Drawing for the job (mm, zero at the part's lowest x, y, z). Give positions to 0.01 mm unless a question says otherwise; leave off trailing zeros. Order: outer loops, then holes, each group sorted by start corner. A loop starts at its lowest first (then second) coordinate and runs counter-clockwise, first axis right, second up. Notation, with made-up numbers: (28.5, -29.75) -> (62.5, -29.75) arc R15 cw to (62.5, -22.75) -> close; hole circle Ø9 at (9.25, 80.5). An arc over 180 degrees is marked (long way). One line per item, written item: value. Start each with the question number.
(1) Saw through at C-C on z = 81.5. Give the cut face in (x, y).
(2) Pin check, flat tips, straight feed: pin 1 (1.5 mm diameter, centred on x = 3.5, y = 12.5, fed in from -Z); pin 2 (1 mm diameter, centred on x = 2.5, y = 5, fed in from +Z); pin 3 (1.5 mm diameter, centred on x = 3, y = 13, fed in from +Z). Stop position of each tip, or through.
(3) Probe line 1 (Z direction, x = 3.25, y = 10.5); line 2 (Y direction, x = 5.25, z = 59.5); line 3 (Z direction, x = 3.5, y = 9.5). List the from-to ranges inside material, lowest first.
(4) Saw through at A-A on x = 3.25. Give the cut face in (y, z).
(5) Saw through at D-D on y = 6.5. Give the cut face in (x, z), plus the area to 3 significant figures.
(6) Saw through at B-B on y = 13.25. Give the cut face in (x, z).
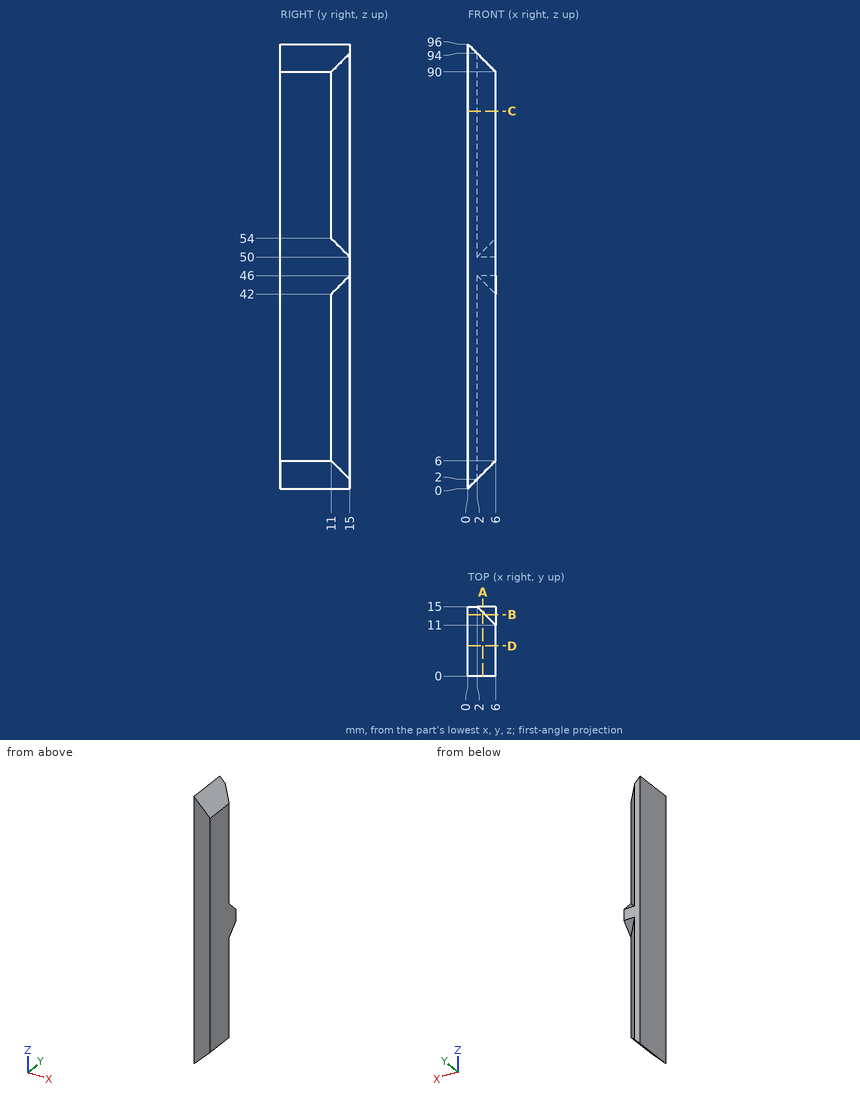
Results below:
1. outline: (0, 0) -> (6, 0) -> (6, 11) -> (2, 15) -> (0, 15) -> close
2. pin 1: stops at z = 2.75
2. pin 2: stops at z = 94
2. pin 3: stops at z = 93.75
3. line 1: z = 3.25 to 92.75
3. line 2: y = 0 to 11.75
3. line 3: z = 3.5 to 92.5
4. outline: (0, 3.25) -> (13.75, 3.25) -> (13.75, 44.75) -> (15, 46) -> (15, 50) -> (13.75, 51.25) -> (13.75, 92.75) -> (0, 92.75) -> close
5. outline: (0, 0) -> (6, 6) -> (6, 90) -> (0, 96) -> close
5. area: 540 mm²
6. outline: (0, 0) -> (3.75, 3.75) -> (3.75, 44.25) -> (6, 44.25) -> (6, 51.75) -> (3.75, 51.75) -> (3.75, 92.25) -> (0, 96) -> close
